The listing builds one solid part. Answer for the finished solid, in the listing's coordinates (mm). A direction names the side the tool comes from. Give positions to 0.01 mm unless a question says otherwise; leave off trailing zeros. Loops run counter-clockwise (first coordinate to the right, second up) from the corner with the lowest first, then second, coordinate; pieces in that order, holes last. Notation, with made-up numbers: M -5.75,-37 L 46.25,-37 A12 cw 46.25,-19 Z; hole C 4.25,35.25 d9. An arc over 180 degrees is marked long. One line per item, written item: value. Start each with the question number.
Q1. A cutting plane is placed at B-B, the plane y = 0. Determine the outline of the cut face in (x, z).
Q2. A cutting plane is placed at C-C, the plane z = -819.5. Determine the outline of the cut face in (x, y), and give its area (3 significant figures).
Q3. Flat-ended cylindrical pins translate along their axes: pin 1 (5 mm diameter, centred on x = -4, y = -15.5, fed in from -Z); pin 2 (12 mm diameter, centred on x = -16, z = -857, fed in from -Y); pin 3 (12 mm diameter, centred on y = -14.5, z = -784, fed in from +X); pin 4 (4.5 mm diameter, centred on y = 16, z = -700.5, fed in from +X). Find the tip coordinate at first contact, or state that the pin passes through.
Q4. Consider L1, parallel to Z at x = 26.5, y = -9; L2, parallel to Y at x = 0.5, z = -794; L3, parallel to X at y = 16, z = -779.5. Determine where each line is inside the solid, lowest interval first.
Q5. For faces 1 (the flat face through (0, 0, -590)), 2 (the flat face through (0, 18.3, -694)), determine the directions among +Z, -Z, +X, -X, +Y, -Y from which every point of the face is accessible in a straight line to the end or side of a thin tool.
Q6. A cutting plane is placed at A-A, the plane x = 0. Determine the outline of the cut face in (y, z).
Q7. A cutting plane is placed at D-D, the plane z = -641.5. Determine the outline of the cut face in (x, y).
from build123d import *
from build123d.topology import SkipClean

# Parameters (mm, degrees)
BOSS_EXTRUDE1_DEPTH = 800
SKETCH3_R           = 30
BOSS_EXTRUDE3_DEPTH = 20
SKETCH4_R           = 30
CUT_EXTRUDE1_DEPTH  = 1391.647331281
SKETCH5_R           = 15
BOSS_EXTRUDE4_DEPTH = 100
CUT_EXTRUDE2_START  = -20
CUT_EXTRUDE2_DEPTH  = 20


with BuildPart() as part:
    # Sketch1 → Boss-Extrude1 (new, symmetric)
    with BuildSketch(Plane.XY):
        with BuildLine():
            Line((-5, 14.142135624), (-5, 18.3))
            Line((-5, 18.3), (5, 18.3))
            Line((5, 18.3), (5, 14.142135624))
            ThreePointArc((5, 14.142135624), (0, -15), (-5, 14.142135624))
        make_face()
    extrude(amount=BOSS_EXTRUDE1_DEPTH, both=True)

    # Sketch3 → Boss-Extrude3 (add)
    with BuildSketch(Plane(origin=(0, 0, 590), x_dir=(-1, 0, 0), z_dir=(0, 0, -1))):
        Circle(SKETCH3_R)
    boss_extrude3 = extrude(amount=-BOSS_EXTRUDE3_DEPTH)

    # Mirror2: Boss-Extrude3 across plane
    add(boss_extrude3.mirror(Plane.XY))

    # Sketch4 → Cut-Extrude1 (cut, through all)
    with BuildSketch(Plane.XY.offset(-590)):
        with Locations(Location((0, 0, 0), (0, 0, 180))):
            Circle(SKETCH4_R)
    extrude(amount=CUT_EXTRUDE1_DEPTH, mode=Mode.SUBTRACT)

    # Sketch5 → Boss-Extrude4 (add)
    with BuildSketch(Plane(origin=(0, 0, -800), x_dir=(-1, 0, 0), z_dir=(0, 0, -1))):
        Circle(SKETCH5_R)
    extrude(amount=BOSS_EXTRUDE4_DEPTH)

    # Sketch6 → Cut-Extrude2 (cut)
    with SkipClean():  # the faces are left unmerged after this step: merging them gives an invalid solid
        with BuildSketch(Plane(origin=(0, 0, -800), x_dir=(-1, 0, 0), z_dir=(0, 0, -1)).offset(CUT_EXTRUDE2_START)):
            with BuildLine():
                Line((5, 14.142135624), (5, 18.3))
                Line((5, 18.3), (-5, 18.3))
                Line((-5, 18.3), (-5, 14.142135624))
                ThreePointArc((-5, 14.142135624), (0, 15), (5, 14.142135624))
            make_face()
        extrude(amount=CUT_EXTRUDE2_DEPTH, mode=Mode.SUBTRACT)


solid = part.part
Answer block:
1. outline: M -30,-610 L -15,-610 L -15,-900 L 15,-900 L 15,-610 L 30,-610 L 30,-590 L -30,-590 Z
2. outline: C 0,0 d30
2. area: 707 mm^2
3. pin 1: z = -900
3. pin 2: y = -11.18
3. pin 3: x = 12.36
3. pin 4: x = 5.99
4. L1: -610 to -590
4. L2: -14.99 to 14.99
4. L3: -5 to 5
5. face 1: +Z, +X, -X, +Y, -Y
5. face 2: -Z, +X, -X, +Y
6. outline: M -30,-610 L -15,-610 L -15,-900 L 15,-900 L 15,-780 L 18.3,-780 L 18.3,-610 L 30,-610 L 30,-590 L -30,-590 Z
7. outline: M -5,14.14 A15 ccw long 5,14.14 L 5,18.3 L -5,18.3 Z
